from build123d import *

# Parameters (mm, degrees)
F0_W     = 40
F0_H     = 37.3
F0_W_2   = 36
F0_H_2   = 33.3
F1_DEPTH = 6.3
F2_DEPTH = 2
F3_R     = 4.5
F4_R     = 1


with BuildPart() as f1:
    # F0 (on Top) → F1 (new body)
    with BuildSketch(Plane.XY):
        Rectangle(F0_W, F0_H)
        Rectangle(F0_W_2, F0_H_2, mode=Mode.SUBTRACT)
    extrude(amount=F1_DEPTH)

    # F0 (on Top) → F2 (join)
    with BuildSketch(Plane.XY):
        Rectangle(F0_W_2, F0_H_2)
    extrude(amount=F2_DEPTH)

    # F3
    f3_edges = [f1.edges().sort_by_distance(p)[0] for p in [
        (-18, 16.65, 4.15),
        (18, 16.65, 4.15),
        (18, -16.65, 4.15),
        (-18, -16.65, 4.15),
        (-20, -18.65, 3.15),
        (20, -18.65, 3.15),
        (20, 18.65, 3.15),
        (-20, 18.65, 3.15),
    ]]
    fillet(f3_edges, radius=F3_R)

    # F4
    f4_edges = [f1.edges().sort_by_distance(p)[0] for p in [
        (0, -18.65, 0),
    ]]
    fillet(f4_edges, radius=F4_R)


solid = f1.part
Read the model definition and answer for the solid it produces. Units are mm, in the model's axes. A direction names the side the tool comes from. Give positions to 0.01 mm unless a question says otherwise; leave off trailing zeros. Write each loop counter-clockwise with the first axis right and the second up, starting at its lowest first coordinate (ties: lowest second). Pieces come first, ordered by that corner, then holes. Notation, with made-up numbers: (27, 73) - (58, 73) arc R17 cw to (58, 80) - close; hole circle Ø7 at (35.25, 24.25). An arc over 180 degrees is marked (long way). Return JSON: item names as keys, results as strings.
Q1. A cutting plane is placed at C-C, the plane z = 4.5. Determine the outline of the cut face in (x, y), and give its area (3 significant figures).
Reply:
{"outline": "(-20, -14.15) arc R4.5 ccw to (-15.5, -18.65) - (15.5, -18.65) arc R4.5 ccw to (20, -14.15) - (20, 14.15) arc R4.5 ccw to (15.5, 18.65) - (-15.5, 18.65) arc R4.5 ccw to (-20, 14.15) - close; hole (-18, -12.15) arc R4.5 ccw to (-13.5, -16.65) - (13.5, -16.65) arc R4.5 ccw to (18, -12.15) - (18, 12.15) arc R4.5 ccw to (13.5, 16.65) - (-13.5, 16.65) arc R4.5 ccw to (-18, 12.15) - close", "area": "293 mm²"}
Q2. A cutting plane is placed at B-B, the plane x = -5.5. Determine the outline of the cut face in (y, z), and give its area (3 significant figures).
Reply:
{"outline": "(-18.65, 1) arc R1 ccw to (-17.65, 0) - (17.65, 0) arc R1 ccw to (18.65, 1) - (18.65, 6.3) - (16.65, 6.3) - (16.65, 2) - (-16.65, 2) - (-16.65, 6.3) - (-18.65, 6.3) - close", "area": "91.4 mm²"}
Q3. A cutting plane is placed at A-A, the plane y = -10. Determine the outline of the cut face in (x, z).
Reply:
{"outline": "(-20, 1) arc R1 ccw to (-19, 0) - (19, 0) arc R1 ccw to (20, 1) - (20, 6.3) - (18, 6.3) - (18, 2) - (-18, 2) - (-18, 6.3) - (-20, 6.3) - close"}
Q4. For a pull along X with two mould halves and no side action, classify faces 1 (the face through (-20, 0, 4)), 2 (the face through (0.217, -18.349, 0.285)), 3 (the face through (18, 0, 4)), 4 (the face through (19.699, 0.198, 0.285)) as released by +X, released by -X, zero draft, split by the parting line, or undercut.
Reply:
{"face 1": "released by -X", "face 2": "zero draft", "face 3": "undercut", "face 4": "released by +X"}
Q5. Given P1, Ø16.5, axis at x = -4, y = -7, coming from the +Z side, flat-ended and moving along its own axis, determine where the tip first touches the part or whether it passes through.
Reply:
{"P1": "z = 2"}
Q6. For faces 5 (the face through (-16.647, 15.367, 4.18)), 6 (the face through (-0.217, 18.349, 0.285)), determine the directions among +Z, -Z, +X, -X, +Y, -Y from which every point of the face is accessible in a straight line to the end or side of a thin tool.
Reply:
{"face 5": "+Z", "face 6": "-Z, +X, -X, +Y"}
Q7. Consider line 1 along X through (y, z) = (-1, 4.25); line 2 along Y through (x, z) = (-12, 4.75); line 3 along Z through (x, y) = (13, 16). Determine where each line is inside the solid, lowest interval first. Write a range as [from, to].
Reply:
{"line 1": "[-20, -18], [18, 20]", "line 2": "[-18.65, -16.65], [16.65, 18.65]", "line 3": "[0, 2]"}
